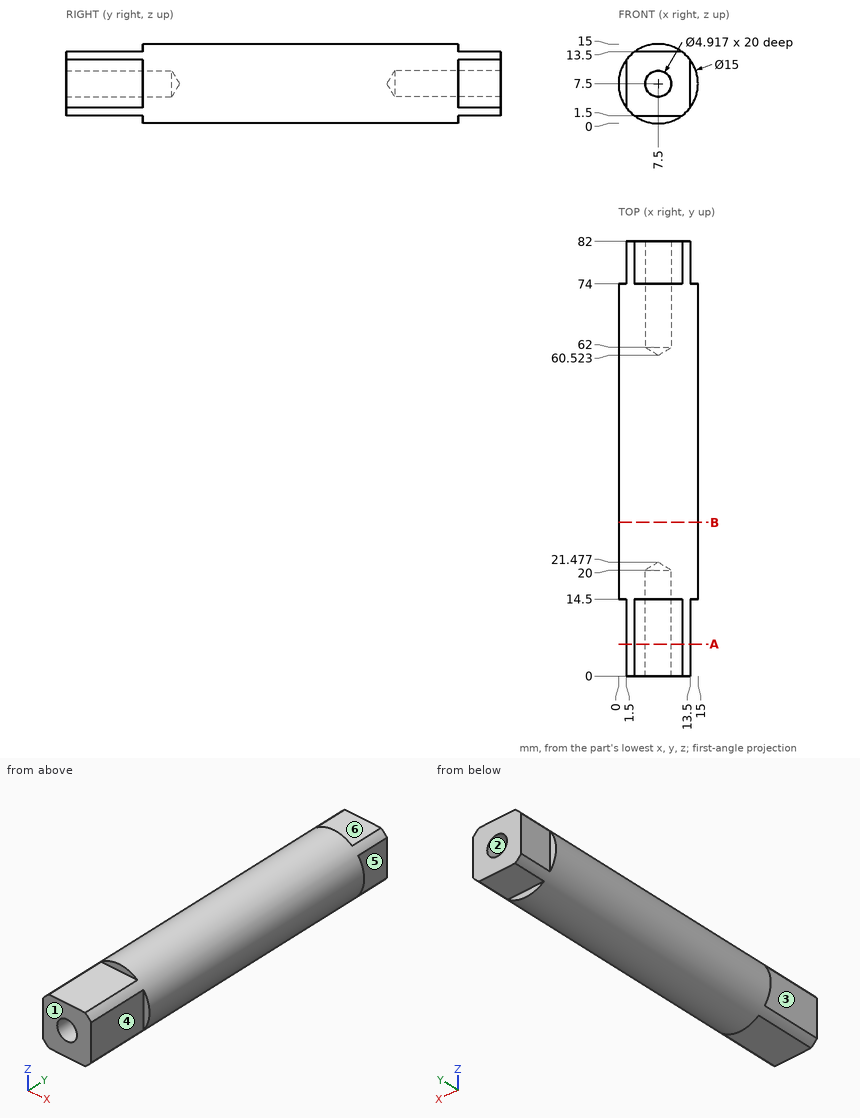
Geometry: see drawing. Coordinates: mm, zero at the bounding-box minimum. A direction names the side the tool comes from. Round coordinates to 2 decimals unless told otherwise and drop trailing zeros. Write each loop counter-clockwise with the first axis right and the second up, starting at its lowest first coordinate (ties: lowest second). Pieces come first, ordered by that corner, then holes.
1) Ray query, L1, parallel to X at y = 72.75, z = 7.5; L2, parallel to Z at x = 7.5, y = 75.25. Return the intervals inside material, ascending.
2) Contact query for flat-ended pins moving along their axis: P1, Ø7, axis at x = 7.5, y = 5.5, coming from the -Z side; P2, Ø1, axis at x = 3.5, y = 70, coming from the +Z side; P3, Ø2.5, axis at x = 9.5, y = 6.5, coming from the +Z side. Output: stop coordinate, or through.
3) Draft query along X for the marked faces 1, 2 and 3. Return one class per face: pulls with the +X half, pulls with the -X half, needs draft (parallel to the pull), parting line crosses it, or undercut.
4) Cut plane B-B (y = 29). Return the cut outline in (x, z), then the cut area to 3 significant figures.
5) Reachability of the marked faces 4, 5 and 6 from +Z, -Z, +X, -X, +Y, -Y: full face, straight path, thin tool, end or side. Return the list, or none.
6) Cut plane A-A (y = 6). Return the cut outline in (x, z), then the cut area to 3 significant figures.
Geometry says:
1. L1: x = 0 to 5.04, 9.96 to 15
1. L2: z = 1.5 to 5.04, 9.96 to 13.5
2. P1: stops at z = 1.5
2. P2: stops at z = 14.13
2. P3: stops at z = 13.5
3. face 1: needs draft
3. face 2: undercut
3. face 3: pulls with the -X half
4. outline: circle Ø15 at (7.5, 7.5)
4. area: 177 mm2
5. face 4: +Z, -Z, +X, -Y
5. face 5: +Z, -Z, +X, +Y
5. face 6: +Z, +X, -X, +Y
6. outline: (1.5, 3) arc R7.5 ccw to (3, 1.5) - (12, 1.5) arc R7.5 ccw to (13.5, 3) - (13.5, 12) arc R7.5 ccw to (12, 13.5) - (3, 13.5) arc R7.5 ccw to (1.5, 12) - close; hole circle Ø4.92 at (7.5, 7.5)
6. area: 121 mm2
